Can you work these out from the model? Positions are in its coordinate system, mm. A direction names the side the tool comes from. Give positions to 0.01 mm unless a question says otherwise; leave off trailing zeros. Loops run counter-clockwise (first coordinate to the right, second up) from the corner with the lowest first, then second, coordinate; pieces in that order, holes last. Notation, with made-up numbers: M 70,68.25 L 81,68.25 A12 cw 81,82.25 Z; hole C 24.5,6.25 d3. An arc over 180 degrees is marked long. One line per item, written item: value. Start each with the question number.
Autodesk Inventor part; units mm, degrees
ref_plane "YZ Plane" through (0, 0, 0) normal (1, 0, 0) x (0, 1, 0)
ref_plane "XZ Plane" through (0, 0, 0) normal (0, 1, 0) x (-1, 0, 0)
ref_plane "XY Plane" through (0, 0, 0) normal (0, 0, 1) x (1, 0, 0)
sketch "Sketch8" plane through (0, 0, 0) normal (0, 0, 1) x (1, 0, 0)
  line L0 (-41.5, -23.5) -> (41.5, -23.5)
  line L1 (41.5, -23.5) -> (41.5, 23.5)
  line L2 (41.5, 23.5) -> (-41.5, 23.5)
  line L3 (-41.5, 23.5) -> (-41.5, -23.5)
  line L4 (-41.5, -23.5) -> (41.5, 23.5) construction
  line L5 (41.5, -23.5) -> (-41.5, 23.5) construction
  point P0 (0, 0)
  dimension "d31" = 47
  dimension "d32" = 83
extrude "Extrusion6" add sketch "Sketch8" against normal blind 32
sketch "Sketch9" plane through (0, 0, 0) normal (0, 0, 1) x (1, 0, 0)
  line L0 (-41.5, -23.5) -> (-41.5, 23.5) construction
  line L1 (-41.5, 0) -> (41.5, 0) construction
  line L2 (41.5, 23.5) -> (41.5, -23.5) construction
  line L3 (-34, -16.5) -> (-9, -16.5)
  line L4 (-9, -16.5) -> (-9, 16.5)
  line L5 (-9, 16.5) -> (-34, 16.5)
  line L6 (-34, 16.5) -> (-34, -16.5)
  line L7 (-34, -16.5) -> (-9, 16.5) construction
  line L8 (-9, -16.5) -> (-34, 16.5) construction
  point P0 (0, 0)
  point P1 (-21.5, 0)
  point P2 (-21.5, 0)
  dimension "d35" = 20
  dimension "d36" = 25
  dimension "d37" = 33
extrude "Extrusion7" add sketch "Sketch9" along normal blind 7
sketch "Sketch10" plane through (0, 0, 7) normal (0, 0, 1) x (1, 0, 0)
  line L0 (-34, -16.5) -> (-34, 16.5) construction
  line L1 (-34, 0) -> (-9, 0) construction
  line L2 (-9, 16.5) -> (-9, -16.5) construction
  line L3 (-24.625, -7) -> (-18.375, -7)
  line L4 (-18.375, -7) -> (-18.375, 7)
  line L5 (-18.375, 7) -> (-24.625, 7)
  line L6 (-24.625, 7) -> (-24.625, -7)
  line L7 (-24.625, -7) -> (-18.375, 7) construction
  line L8 (-18.375, -7) -> (-24.625, 7) construction
  line L9 (-41.5, 23.5) -> (-41.5, -23.5)
  point P0 (0, 0)
  point P1 (-21.5, 0)
  point P2 (-21.5, 0)
  dimension "d40" = 20
  dimension "d41" = 14
  dimension "d42" = 6.25
extrude "Extrusion8" add sketch "Sketch10" along normal blind 18.28
equation "\"d31\" = poeWidth"
equation "\"d32\" = poeLength"
equation "\"d33\" = poeMajorDepth"
equation "\"d36\" = plugBaseLength"
equation "\"d37\" = plugBaseWidth"
equation "\"d38\" = plugBaseDepth"
equation "\"d41\" = plugWidth"
equation "\"d42\" = plugLength"
equation "\"d43\" = plugDepth"
equation "\"poeLength\" = 83"
equation "\"poeWidth\" = 47"
equation "\"poeMajorDepth\" = 32"
equation "\"plugBaseWidth\" = 33"
equation "\"plugBaseLength\" = 25"
equation "\"plugBaseDepth\" = 7"
equation "\"plugBaseCenterFromTop\" = 20"
equation "\"plugWidth\" = 14"
equation "\"plugLength\" = 6.25"
equation "\"plugDepth\" = 18.28"
equation "\"plugCenterFromTop\" = 20"
properties part number "poeAdapter" material "PC/ABS Plastic"
Q1. I need wall thicknesses on line 1 along Z through (x, y) = (-20, 16); line 2 along Z through (x, y) = (8.5, 13.5); line 3 along Y through (x, z) = (-16, 4). Which ranges of each line are inside material? Lowest first, please.
Q2. If we section it at C-C, the plane z = 15.5: Write out the boundary of the cut face in (x, y) (3 decimals), plus the area to 3 significant figures.
Q3. If we section it at A-A, the plane y = -8.5: Write out the boundary of the cut face in (x, z), plus the area to 3 significant figures.
Q4. If we section it at D-D, the plane x = 11: Write out the boundary of the cut face in (y, z), plus the area to 3 significant figures.
Q5. For P1, Ø15.5, axis at y = -3, z = 20, coming from the -X side (3 decimals); P2, Ø1, axis at x = 9.5, y = -4, coming from the +Z side; P3, Ø7.5, axis at x = -17, z = 2, coming from the +Y side; P4, Ø2, axis at y = -5.5, z = 5, coming from the -X side, each with a flat end and sliding along its axis, tell me the tip position at first contact or that it passes through.
Q6. Which directions (+Z, -Z, +X, -X, +Y, -Y) give clear straight access to the entire face, cutting with the end or side of a thin tool? Please do faces 1 (the face through (-24.625, 0, 16)), 2 (the face through (-18.375, 0, 16)), 3 (the face through (-22, -16.5, 3)), 4 (the face through (-21, 16.5, 3)).
Q7. If we section it at B-B, the plane x = -23: Write out the boundary of the cut face in (y, z).
Response:
1. line 1: -32 to 7
1. line 2: -32 to 0
1. line 3: -16.5 to 16.5
2. outline: M -24.625,-7 L -18.375,-7 L -18.375,7 L -24.625,7 Z
2. area: 87.5 mm^2
3. outline: M -41.5,-32 L 41.5,-32 L 41.5,0 L -9,0 L -9,7 L -34,7 L -34,0 L -41.5,0 Z
3. area: 2,830 mm^2
4. outline: M -23.5,-32 L 23.5,-32 L 23.5,0 L -23.5,0 Z
4. area: 1,500 mm^2
5. P1: x = -24.625
5. P2: z = 0
5. P3: y = 23.5
5. P4: x = -34
6. face 1: +Z, -X, +Y, -Y
6. face 2: +Z, +X, +Y, -Y
6. face 3: +Z, +X, -X, -Y
6. face 4: +Z, +X, -X, +Y
7. outline: M -23.5,-32 L 23.5,-32 L 23.5,0 L 16.5,0 L 16.5,7 L 7,7 L 7,25.28 L -7,25.28 L -7,7 L -16.5,7 L -16.5,0 L -23.5,0 Z
